from build123d import *

# Parameters (mm, degrees)
SKETCH1_W                       = 609.6
SKETCH1_H                       = 200.025
BOSS_EXTRUDE1_DEPTH             = 6.35
F_1_4_0_25_DIAMETER_SLOT1_DEPTH = 6.35
CUT_EXTRUDE1_DEPTH              = 321.85177677


# Read off the part's stored shape, not the designer's step: 1/4 (0.25) Diameter Slot1
with BuildPart() as part:
    # Sketch1 → Boss-Extrude1 (new body)
    with BuildSketch(Plane.XY):
        Rectangle(SKETCH1_W, SKETCH1_H)
    extrude(amount=BOSS_EXTRUDE1_DEPTH)

    # 1/4 (0.25) Diameter Slot1 outline → 1/4 (0.25) Diameter Slot1 (cut)
    with BuildSketch(Plane.XY):
        with BuildLine():
            Line((219.075, -58.7375), (225.425, -58.7375))
            ThreePointArc((225.425, -58.7375), (228.6, -55.5625), (225.425, -52.3875))
            Line((225.425, -52.3875), (219.075, -52.3875))
            ThreePointArc((219.075, -52.3875), (215.9, -55.5625), (219.075, -58.7375))
        make_face()
        with BuildLine():
            ThreePointArc((-219.075, -58.7375), (-215.9, -55.5625), (-219.075, -52.3875))
            Line((-219.075, -52.3875), (-225.425, -52.3875))
            ThreePointArc((-225.425, -52.3875), (-228.6, -55.5625), (-225.425, -58.7375))
            Line((-225.425, -58.7375), (-219.075, -58.7375))
        make_face()
        with BuildLine():
            ThreePointArc((276.225, -58.7375), (279.4, -55.5625), (276.225, -52.3875))
            Line((276.225, -52.3875), (269.875, -52.3875))
            ThreePointArc((269.875, -52.3875), (266.7, -55.5625), (269.875, -58.7375))
            Line((269.875, -58.7375), (276.225, -58.7375))
        make_face()
        with BuildLine():
            ThreePointArc((-269.875, -58.7375), (-266.7, -55.5625), (-269.875, -52.3875))
            Line((-269.875, -52.3875), (-276.225, -52.3875))
            ThreePointArc((-276.225, -52.3875), (-279.4, -55.5625), (-276.225, -58.7375))
            Line((-276.225, -58.7375), (-269.875, -58.7375))
        make_face()
        with BuildLine():
            Line((219.075, 52.3875), (225.425, 52.3875))
            ThreePointArc((225.425, 52.3875), (228.6, 55.5625), (225.425, 58.7375))
            Line((225.425, 58.7375), (219.075, 58.7375))
            ThreePointArc((219.075, 58.7375), (215.9, 55.5625), (219.075, 52.3875))
        make_face()
        with BuildLine():
            ThreePointArc((-219.075, 52.3875), (-215.9, 55.5625), (-219.075, 58.7375))
            Line((-219.075, 58.7375), (-225.425, 58.7375))
            ThreePointArc((-225.425, 58.7375), (-228.6, 55.5625), (-225.425, 52.3875))
            Line((-225.425, 52.3875), (-219.075, 52.3875))
        make_face()
        with BuildLine():
            ThreePointArc((276.225, 52.3875), (279.4, 55.5625), (276.225, 58.7375))
            Line((276.225, 58.7375), (269.875, 58.7375))
            ThreePointArc((269.875, 58.7375), (266.7, 55.5625), (269.875, 52.3875))
            Line((269.875, 52.3875), (276.225, 52.3875))
        make_face()
        with BuildLine():
            ThreePointArc((-269.875, 52.3875), (-266.7, 55.5625), (-269.875, 58.7375))
            Line((-269.875, 58.7375), (-276.225, 58.7375))
            ThreePointArc((-276.225, 58.7375), (-279.4, 55.5625), (-276.225, 52.3875))
            Line((-276.225, 52.3875), (-269.875, 52.3875))
        make_face()
    extrude(amount=F_1_4_0_25_DIAMETER_SLOT1_DEPTH, mode=Mode.SUBTRACT)

    # Sketch4 → Cut-Extrude1 (cut, through all)
    with BuildSketch(Plane.XY.offset(6.35)):
        with BuildLine():
            Line((-98.425, -100.0125), (-3.540889475, -72.46550017))
            ThreePointArc((-3.540889475, -72.46550017), (0, -71.96189725), (3.540889475, -72.46550017))
            Line((3.540889475, -72.46550017), (98.425, -100.0125))
            Line((98.425, -100.0125), (-98.425, -100.0125))
        make_face()
    extrude(amount=-CUT_EXTRUDE1_DEPTH, mode=Mode.SUBTRACT)


solid = part.part
Input: part model. Units: mm. Frame: model coordinates. A direction names the side the tool comes from. Coordinates: 2 decimals unless noted, no trailing zeros. Order: outer loops, then holes, each group sorted by start corner. A loop starts at its lowest first (then second) coordinate and runs counter-clockwise, first axis right, second up.
1. Cut plane B-B, the plane x = 87.5. Return loops of the section in (y, z).
Checked values:
outline: (-96.84, 0) - (100.01, 0) - (100.01, 6.35) - (-96.84, 6.35) - close
2. Cut plane C-C, the plane x = -79. Return loops of the section in (y, z), plus the area to 3 significant figures.
Checked values:
outline: (-94.37, 0) - (100.01, 0) - (100.01, 6.35) - (-94.37, 6.35) - close
area: 1,230 mm2
3. Cut plane A-A, the plane z = 2.5. Count the separate pieces of the cut face and the enclosed holes in it, plus the area to 3 significant figures.
Checked values:
separate pieces: 1
enclosed holes: 8
area: 119,000 mm2
4. Ray query, line 1 along X through (y, z) = (-55, 6); line 2 along Y through (x, z) = (-225.5, 5.5); line 3 along Y through (x, z) = (-269, 3). Return the intervals inside material, ascending.
Checked values:
line 1: x = -304.8 to -279.35, -266.75 to -228.55, -215.95 to 215.95, 228.55 to 266.75, 279.35 to 304.8
line 2: y = -100.01 to -58.74, -52.39 to 52.39, 58.74 to 100.01
line 3: y = -100.01 to -58.61, -52.51 to 52.51, 58.61 to 100.01
5. Draft query along Y for faces 3 (the flat face through (-51.647, -86.432, 3.219)), 4 (the flat face through (-4, 1, 0)). Return one class per face: +Y half, -Y half, draft (parallel to the pull), parting line (faces both ways), or undercut.
Checked values:
face 3: -Y half
face 4: draft
6. Access query for faces 1 (the flat face through (-4, 1, 6.35)), 2 (the flat face through (50.319, -86.046, 3.219)). Directions: +Z, -Z, +X, -X, +Y, -Y. A direction counts if a zero-diameter tool reaches every point of the face in a straight line with its end or side. Return the directions, or none.
Checked values:
face 1: +Z, +X, -X, +Y, -Y
face 2: +Z, -Z, -Y
